The model under review builds one solid part; all positions refer to its coordinate system, in mm. Face numbers are marked on the shaded views. A direction names the side the tool comes from. Coordinates: 2 decimals unless noted, no trailing zeros. Order: outer loops, then holes, each group sorted by start corner. A loop starts at its lowest first (then second) coordinate and runs counter-clockwise, first axis right, second up. Notation, with made-up numbers: M 38,65 L 70,65 A12 ccw 70,76 Z; hole C 24.5,68 d3. An arc over 180 degrees is marked long. One line per item, written item: value.
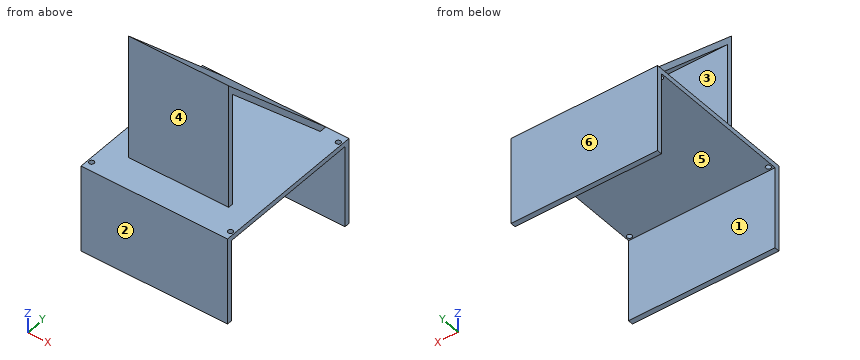
```python
from build123d import *

# Parameters (mm, degrees)
SKIZZE1_W                       = 117
SKIZZE1_H                       = 125
AUFSATZ_LINEAR_AUSTRAGEN1_DEPTH = 4
SKIZZE2_W                       = 80
SKIZZE2_H                       = 100
AUFSATZ_LINEAR_AUSTRAGEN2_DEPTH = 100
SCHNITT_LINEAR_AUSTRAGEN1_DEPTH = 100
SCHNITT_LINEAR_AUSTRAGEN2_DEPTH = 100
SKIZZE5_W                       = 117
SKIZZE5_H                       = 4
AUFSATZ_LINEAR_AUSTRAGEN3_DEPTH = 66
SKIZZE6_R                       = 2
SCHNITT_LINEAR_AUSTRAGEN3_DEPTH = 70


with BuildPart() as part:
    # Skizze1 → Aufsatz-Linear austragen1 (new body)
    with BuildSketch(Plane.XY):
        with Locations((58.5, 62.5)):
            Rectangle(SKIZZE1_W, SKIZZE1_H)
    extrude(amount=AUFSATZ_LINEAR_AUSTRAGEN1_DEPTH)

    # Skizze2 → Aufsatz-Linear austragen2 (add)
    with BuildSketch(Plane.XY.offset(4)):
        with Locations((58.5, 75)):
            Rectangle(SKIZZE2_W, SKIZZE2_H)
    extrude(amount=AUFSATZ_LINEAR_AUSTRAGEN2_DEPTH)

    # Skizze3 → Schnitt-Linear austragen1 (cut)
    with BuildSketch(Plane.ZY.offset(-18.5)):
        Polygon((104, 25), (104, 125), (4, 125), align=None)
    extrude(amount=-SCHNITT_LINEAR_AUSTRAGEN1_DEPTH, mode=Mode.SUBTRACT)

    # Skizze4 → Schnitt-Linear austragen2 (cut)
    with BuildSketch(Plane.ZY.offset(-18.5)):
        Polygon((4, 119.343145751), (94.343145751, 29), (4, 29), align=None)
    extrude(amount=-SCHNITT_LINEAR_AUSTRAGEN2_DEPTH, mode=Mode.SUBTRACT)

    # Skizze5 → Aufsatz-Linear austragen3 (add)
    with BuildSketch(Plane(origin=(0, 0, 0), x_dir=(-1, 0, 0), z_dir=(0, 0, -1))):
        with Locations((-58.5, 123)):
            Rectangle(SKIZZE5_W, SKIZZE5_H)
        with Locations((-58.5, 2)):
            Rectangle(SKIZZE5_W, SKIZZE5_H)
    extrude(amount=AUFSATZ_LINEAR_AUSTRAGEN3_DEPTH)

    # Skizze6 → Schnitt-Linear austragen3 (cut)
    with BuildSketch(Plane(origin=(0, 0, 0), x_dir=(-1, 0, 0), z_dir=(0, 0, -1))):
        with Locations((-114, 118)):
            Circle(SKIZZE6_R)
        with Locations((-3, 118)):
            Circle(SKIZZE6_R)
        with Locations((-3, 7)):
            Circle(SKIZZE6_R)
        with Locations((-114, 7)):
            Circle(SKIZZE6_R)
    extrude(amount=-SCHNITT_LINEAR_AUSTRAGEN3_DEPTH, mode=Mode.SUBTRACT)


solid = part.part
```
(1) We need section C-C, the plane y = 7. State the section outline as (x, z) points.
Geometry results:
outline: M 0,0 L 1,0 L 1,4 L 0,4 Z; M 5,0 L 112,0 L 112,4 L 5,4 Z; M 116,0 L 117,0 L 117,4 L 116,4 Z
(2) We need section B-B, the plane x = 114. State the section outline as (y, z) points.
Geometry results:
outline: M 0,-66 L 4,-66 L 4,0 L 5,0 L 5,4 L 0,4 Z; M 9,0 L 116,0 L 116,4 L 9,4 Z; M 120,0 L 121,0 L 121,-66 L 125,-66 L 125,4 L 120,4 Z
(3) For L1, parallel to Y at x = 114, z = 2.9; L2, parallel to Y at x = 39.5, z = -25; L3, parallel to Z at x = 7, y = 59.5, list the stretches that pass through material, from the lowest coordinate up.
Geometry results:
L1: y = 0 to 5, 9 to 116, 120 to 125
L2: y = 0 to 4, 121 to 125
L3: z = 0 to 4
(4) Insertion check: pin 1 Ø2 at (x, z) = (96.5, 36.5) entering from +Y; pin 2 Ø3 at (x, y) = (3, 7) entering from +Z; pin 3 Ø2 at (x, y) = (74.5, 40.5) entering from -Z; pin 4 Ø4 at (x, z) = (19, 47.5) entering from +Y. Each pin has a flat end and moves straight along its axis. Give the tip position at first contact, or say it passes through.
Geometry results:
pin 1: stops at y = 93.5
pin 2: passes through
pin 3: stops at z = 0
pin 4: stops at y = 83.5
(5) We need section D-D, the plane x = 45.5. State the section outline as (y, z) points, plus the area to 3 significant figures.
Geometry results:
outline: M 0,-66 L 4,-66 L 4,0 L 121,0 L 121,-66 L 125,-66 L 125,4 L 25,104 L 25,4 L 0,4 Z; hole M 29,4 L 119.34,4 L 29,94.34 Z
area: 1,950 mm2
(6) We need section A-A, the plane z = -40. State the section outline as (x, y) points.
Geometry results:
outline: M 0,0 L 117,0 L 117,4 L 0,4 Z; M 0,121 L 117,121 L 117,125 L 0,125 Z
(7) Tool access review of the marked faces 1, 2 and 3: name each direction out of +Z, -Z, +X, -X, +Y, -Y from which nothing blocks a thin tool from reaching the whole face with its end or side.
Geometry results:
face 1: -Z, +X, -X
face 2: +Z, -Z, +X, -X, -Y
face 3: +X, -X
(8) Mouldability with a two-part tool opening along Y and no side actions: class the marked faces 4, 5 and 6 as +Y half, -Y half, draft (parallel to the pull), parting line (faces both ways), or undercut.
Geometry results:
face 4: -Y half
face 5: undercut
face 6: +Y half
